Source: CAD feature listing. Evaluate the final solid. Frame: model axes, mm. Coordinates: 2 decimals unless noted, no trailing zeros. Order: outer loops, then holes, each group sorted by start corner. A loop starts at its lowest first (then second) coordinate and runs counter-clockwise, first axis right, second up.
```python
from build123d import *

# Parameters (mm, degrees)
SKETCH1_W           = 5
SKETCH1_H           = 15
BOSS_EXTRUDE1_DEPTH = 5


with BuildPart() as part:
    # Sketch1 → Boss-Extrude1 (new body)
    with BuildSketch(Plane.XY):
        Polygon((885, 50), (0, 50), (0, 36.209811371), (-5, 36.209811371), (-5, 11.209811371), (0, 11.209811371), (0, -5), (20, -5), (20, 0), (70, 0), (70, -5), (110, -5), (110, 0), (160, 0), (160, -5), (200, -5), (200, 0), (250, 0), (250, -5), (290, -5), (290, 0), (340, 0), (340, -5), (380, -5), (380, 0), (430, 0), (430, -5), (470, -5), (470, 0), (520, 0), (520, -5), (560, -5), (560, 0), (610, 0), (610, -5), (650, -5), (650, 0), (700, 0), (700, -5), (740, -5), (740, 0), (790, 0), (790, -5), (830, -5), (830, 0), (885, 0), (885, 5), (900, 5), (900, 20), (885, 20), (885, 30), (900, 30), (900, 45), (885, 45), align=None)
        with Locations((12.5, 12.5)):
            Rectangle(SKETCH1_W, SKETCH1_H, mode=Mode.SUBTRACT)
        with Locations((312.5, 12.5)):
            Rectangle(SKETCH1_W, SKETCH1_H, mode=Mode.SUBTRACT)
        with Locations((612.5, 12.5)):
            Rectangle(SKETCH1_W, SKETCH1_H, mode=Mode.SUBTRACT)
        with Locations((12.5, 37.5)):
            Rectangle(SKETCH1_W, SKETCH1_H, mode=Mode.SUBTRACT)
        with Locations((312.5, 37.5)):
            Rectangle(SKETCH1_W, SKETCH1_H, mode=Mode.SUBTRACT)
        with Locations((612.5, 37.5)):
            Rectangle(SKETCH1_W, SKETCH1_H, mode=Mode.SUBTRACT)
    extrude(amount=-BOSS_EXTRUDE1_DEPTH)


solid = part.part
```
1. Ray query, line 1 (X direction, y = 35, z = -0.2); line 2 (X direction, y = 6.5, z = -4.25); line 3 (X direction, y = 22.5, z = -2.65). Return the intervals inside material, ascending.
Findings:
line 1: x = -5 to 10, 15 to 310, 315 to 610, 615 to 900
line 2: x = 0 to 10, 15 to 310, 315 to 610, 615 to 900
line 3: x = -5 to 885
2. Section query A-A on z = -3.9. Count the separate pieces of the cut face and the enclosed holes in it, plus the area to 3 significant figures.
Findings:
separate pieces: 1
enclosed holes: 6
area: 46,300 mm2
3. Pin query (flat end, axial travel): P1, Ø1.5, axis at y = -0.5, z = -2, coming from the -X side; P2, Ø2.5, axis at x = 233, z = -2.5, coming from the -Y side; P3, Ø2.5, axis at y = -3, z = -3, coming from the +X side. Return the tip coordinate at first contact, or that it passes through.
Findings:
P1: stops at x = 0
P2: stops at y = 0
P3: stops at x = 830
4. Section query B-B on x = 396.5. Return loops of the section in (y, z).
Findings:
outline: (0, -5) - (50, -5) - (50, 0) - (0, 0) - close
